```python
from build123d import *

# Parameters (mm, degrees)
SKETCH1_R           = 10.5
BOSS_EXTRUDE1_DEPTH = 2.3
SKETCH2_R           = 0.75
CUT_EXTRUDE1_DEPTH  = 3.3
SKETCH3_R           = 1.5
CUT_EXTRUDE2_DEPTH  = 2.3
CIRPATTERN1_COUNT   = 4
SKETCH4_R           = 4.4
SKETCH4_R_2         = 2.5
BOSS_EXTRUDE2_DEPTH = 3.2


with BuildPart() as part:
    # Sketch1 → Boss-Extrude1 (new body)
    with BuildSketch(Plane.XY):
        Circle(SKETCH1_R)
    extrude(amount=BOSS_EXTRUDE1_DEPTH)

    # Sketch2 → Cut-Extrude1 (cut, through all)
    with BuildSketch(Plane.XY.offset(2.3)):
        with Locations((0, 7)):
            Circle(SKETCH2_R)
    cut_extrude1 = extrude(amount=-CUT_EXTRUDE1_DEPTH, mode=Mode.SUBTRACT)

    # Sketch3 → Cut-Extrude2 (cut)
    with BuildSketch(Plane.XY.offset(2.3)):
        Circle(SKETCH3_R)
    extrude(amount=-CUT_EXTRUDE2_DEPTH, mode=Mode.SUBTRACT)

    # CirPattern1: Cut-Extrude1 ×4 about axis
    cirpattern1_axis = Axis((0, 0, 0), (0, 0, 1))
    for i in range(1, CIRPATTERN1_COUNT):
        add(cut_extrude1.rotate(cirpattern1_axis, i * 360 / CIRPATTERN1_COUNT), mode=Mode.SUBTRACT)

    # Sketch4 → Boss-Extrude2 (add)
    with BuildSketch(Plane.XY.offset(2.3)):
        Circle(SKETCH4_R)
        Circle(SKETCH4_R_2, mode=Mode.SUBTRACT)
    extrude(amount=BOSS_EXTRUDE2_DEPTH)


solid = part.part
```
Read the model definition and answer for the solid it produces. Units are mm, in the model's axes. A direction names the side the tool comes from. Round coordinates to 2 decimals unless told otherwise and drop trailing zeros. Loops run counter-clockwise (first coordinate to the right, second up) from the corner with the lowest first, then second, coordinate; pieces in that order, holes last. Notation, with made-up numbers: (-33.5, 42) -> (11.5, 42) arc R18 ccw to (11.5, 68) -> close; hole circle Ø7 at (50, -6.75). An arc over 180 degrees is marked (long way). One line per item, written item: value.
1) Flat-ended cylindrical pins translate along their axes: P1, Ø1.2, axis at x = 7, y = 0, coming from the -Z side; P2, Ø2, axis at y = -2.5, z = 2.5, coming from the +X side; P3, Ø1.5, axis at x = -0.5, y = 1, coming from the +Z side; P4, Ø1, axis at x = -0.5, z = 3, coming from the -Y side. Find the tip coordinate at first contact, or state that the pin passes through.
Answer list:
P1: passes through
P2: stops at x = 10.39
P3: stops at z = 2.3
P4: stops at y = -4.4
2) The mould has two halves that part along Y. Classify faces 3 (the face through (10, 3.2, 1.1)), 4 (the face through (2, -2, 5.5)), 5 (the face through (0.163, -6.268, 1.166)): pulls with the +Y half, pulls with the -Y half, needs draft (parallel to the pull), parting line crosses it, or undercut.
Answer list:
face 3: parting line crosses it
face 4: needs draft
face 5: undercut
3) A cutting plane is placed at C-C (y = 7). Determine the outline of the cut face in (x, z).
Answer list:
outline: (-7.83, 0) -> (-0.75, 0) -> (-0.75, 2.3) -> (-7.83, 2.3) -> close; (0.75, 0) -> (7.83, 0) -> (7.83, 2.3) -> (0.75, 2.3) -> close
4) Consider L1, parallel to Y at x = 0, z = 0.9; L2, parallel to Y at x = 0, z = 3.6; L3, parallel to Y at x = -0.5, z = 2.05. Determine where each line is inside the solid, lowest interval first. Write a range as [from, to].
Answer list:
L1: y = [-10.5, -7.75], [-6.25, -1.5], [1.5, 6.25], [7.75, 10.5]
L2: y = [-4.4, -2.5], [2.5, 4.4]
L3: y = [-10.49, -7.56], [-6.44, -1.41], [1.41, 6.44], [7.56, 10.49]
5) For faces 1 (the face through (-0.163, 6.268, 1.166)), 2 (the face through (0, -2, 2.3)), determine the directions among +Z, -Z, +X, -X, +Y, -Y from which every point of the face is accessible in a straight line to the end or side of a thin tool.
Answer list:
face 1: +Z, -Z
face 2: +Z
6) A cutting plane is placed at D-D (x = -7.25). Determine the outline of the cut face in (y, z), and give its area (3 significant figures).
Answer list:
outline: (-7.6, 0) -> (-0.71, 0) -> (-0.71, 2.3) -> (-7.6, 2.3) -> close; (0.71, 0) -> (7.6, 0) -> (7.6, 2.3) -> (0.71, 2.3) -> close
area: 31.7 mm²
7) A cutting plane is placed at A-A (x = 0). Determine the outline of the cut face in (y, z), and give its area (3 significant figures).
Answer list:
outline: (-10.5, 0) -> (-7.75, 0) -> (-7.75, 2.3) -> (-10.5, 2.3) -> close; (-6.25, 0) -> (-1.5, 0) -> (-1.5, 2.3) -> (-2.5, 2.3) -> (-2.5, 5.5) -> (-4.4, 5.5) -> (-4.4, 2.3) -> (-6.25, 2.3) -> close; (1.5, 0) -> (6.25, 0) -> (6.25, 2.3) -> (4.4, 2.3) -> (4.4, 5.5) -> (2.5, 5.5) -> (2.5, 2.3) -> (1.5, 2.3) -> close; (7.75, 0) -> (10.5, 0) -> (10.5, 2.3) -> (7.75, 2.3) -> close
area: 46.7 mm²
